Can you work these out from the model? Positions are in its coordinate system, mm. A direction names the side the tool comes from. Coordinates: 2 decimals unless noted, no trailing zeros. Order: outer loops, then holes, each group sorted by start corner. A loop starts at its lowest first (then second) coordinate and runs counter-clockwise, first axis right, second up. Notation, with made-up numbers: (59, -19) -> (98, -19) arc R22 cw to (98, -7) -> close; hole circle Ø11 at (17, 59). An arc over 180 degrees is marked (long way). Answer in a Markdown table with one row per item. Add a question column.
1. If I drill on line 1 along Y through (x, z) = (5.25, 2.7) (3 decimals); line 2 along Y through (x, z) = (5.75, 2.5); line 3 along X through (y, z) = (65, 2.45), over which ranges is the centre line in solid material (lowest first)? Write a range as [from, to].
2. On a 3-axis mill with a long thin cutter (end or side, diameter ignored), from which of +Z, -Z, +X, -X, +Y, -Y can I reach the whole of each face in a straight line? I mean faces 1 (the face through (7.561, 65.054, 3.507)), 2 (the face through (3.325, 14.513, 2.521)), 3 (the face through (6.8, 64.8, 2)), 4 (the face through (9.86, 13.47, 2.52)), 5 (the face through (6, 39, 4)). Say none if no direction works.
3. We'd pull the mould along X, two halves only. Please class faces 6 (the face through (3.29, 68.42, 3.51)), 7 (the face through (6, 39, 1)), 8 (the face through (11.116, 37.836, 2.479)), 9 (the face through (-0.461, 62.927, 2.521)): pulls with the +X half, pulls with the -X half, needs draft (parallel to the pull), parting line crosses it, or undercut.
4. Imagine slicing it at B-B on y = 50. Write out the boundary of the cut face in (x, z), plus the area to 3 significant figures.
5. Will these pins go through, and if not, where does the flat tip stop? pin 1 (4.5 mm diameter, centred on x = 5.59, y = 11.38, fed in from +Z); pin 2 (1.5 mm diameter, centred on x = 3, y = 43, fed in from -Z); pin 3 (1 mm diameter, centred on x = 2, z = 2, fed in from -Y).
6. Imagine slicing it at A-A on z = 1.55. Write out the boundary of the cut face in (x, y), plus the area to 3 significant figures.
7. Imagine slicing it at C-C on x = 10.5. Write out the boundary of the cut face in (y, z), plus the area to 3 significant figures.
Autodesk Inventor part; units mm, degrees
ref_plane "Work Plane1" through (-0.0405, 69.8618, 0) normal (0, 0, 1) x (0.6413599, 0.7672402, 0)
ref_plane "Work Plane3" through (5.5931, 11.378, 1) normal (0, 0, 1) x (1, 0, 0)
ref_plane "Work Plane6" through (4.3681, 64.2214, 5) normal (0, 0, 1) x (1, 0, 0)
ref_plane "Work Plane1" through (-0.0405, 69.8618, 0) normal (0, 0, 1) x (0.6413599, 0.7672402, 0)
ref_plane "Work Plane3" through (5.5931, 11.378, 1) normal (0, 0, 1) x (1, 0, 0)
sketch "Sketch2" plane through (5.5931, 11.378, 1) normal (0, 0, 1) x (1, 0, 0)
  arc A0 (-2.9323, 0.6339) -> (-4.1247, 52.0744) centre (-110.4489, 23.8756) ccw
  arc A1 (2.9323, -0.6339) -> (1.6748, 53.6125) centre (-110.4489, 23.8756) ccw
  arc A2 (1.6748, 53.6125) -> (-4.1247, 52.0744) centre (-1.225, 52.8435) ccw
  circle A3 centre (0, 0) radius 3
  circle A4 centre (0, 0) radius 1.25
  circle A5 centre (-1.225, 52.8435) radius 3
  circle A6 centre (-1.225, 52.8435) radius 1.4795
  point P0 (-5.5931, -11.378)
  point P1 (-2.9323, 0.6339)
  point P2 (2.9323, -0.6339)
extrude "Extrusion2" add sketch "Sketch2" along normal blind 3
ref_plane "Work Plane6" through (4.3681, 64.2214, 5) normal (0, 0, 1) x (1, 0, 0)
sketch "Sketch4" plane through (4.3681, 64.2214, 4) normal (0, 0, 1) x (1, 0, 0)
  arc A0 (4.1572, -53.4773) -> (2.8997, 0.7691) centre (-109.2239, -28.9678) ccw construction
  arc A1 (-1.7073, -52.2096) -> (-2.8997, -0.7691) centre (-109.2239, -28.9678) ccw construction
  circle A2 centre (0, 0) radius 3 construction
  circle A3 centre (0, 0) radius 3 construction
  circle A4 centre (0, 0) radius 1.4795 construction
  arc A5 (0.2521, -0.9677) -> (-0.2606, 0.9654) centre (-109.2239, -28.9678) ccw construction
  arc A6 (5.0961, 0.2712) -> (4.5608, 2.2899) centre (-109.2239, -28.9678) ccw
  arc A7 (-4.592, -2.2067) -> (-5.082, -0.359) centre (-109.2239, -28.9678) ccw
  arc A8 (-4.592, -2.2067) -> (5.0961, 0.2712) centre (0.2521, -0.9677) ccw
  arc A9 (4.5608, 2.2899) -> (-5.082, -0.359) centre (-0.2606, 0.9654) ccw
  arc A10 (-1.7073, -52.2096) -> (4.1572, -53.4773) centre (1.225, -52.8435) ccw
  arc A11 (2.8997, 0.7691) -> (-2.8997, -0.7691) centre (0, 0) ccw
  arc A12 (-1.7073, -52.2096) -> (-2.8997, -0.7691) centre (-109.2239, -28.9678) ccw
  point P0 (-4.3681, -64.2214)
  dimension "d16" = 10
  dimension "d26" = 1
  dimension "d27" = 1
extrude "Extrusion4" add sketch "Sketch4" against normal blind 3
ref_plane "Work Plane7" through (5.5931, 11.378, 5) normal (0, 0, 1) x (1, 0, 0)
sketch "Sketch5" plane through (5.5931, 11.378, 5) normal (0, 0, 1) x (1, 0, 0)
  arc A0 (-0.9646, 51.8435) -> (-1.4951, 53.8435) centre (-110.4489, 23.8756) ccw construction
  arc A1 (0.7309, 52.2766) -> (0.1923, 54.3076) centre (-110.4489, 23.8756) ccw
  arc A2 (-2.6602, 51.4103) -> (-3.1824, 53.3794) centre (-110.4489, 23.8756) ccw
  arc A3 (-2.6602, 51.4103) -> (0.7309, 52.2766) centre (-0.9646, 51.8435) ccw
  arc A4 (0.1923, 54.3076) -> (-3.1824, 53.3794) centre (-1.4951, 53.8435) ccw
  arc A5 (2.6687, 52.7716) -> (2.1206, 54.838) centre (-110.4489, 23.8756) ccw
  arc A6 (2.1206, 54.838) -> (-5.1108, 52.849) centre (-1.4951, 53.8435) ccw
  arc A7 (-4.598, 50.9153) -> (-5.1108, 52.849) centre (-110.4489, 23.8756) ccw
  arc A8 (-4.598, 50.9153) -> (2.6687, 52.7716) centre (-0.9646, 51.8435) ccw
  arc A9 (3.3358, 55.1334) -> (-6.307, 52.4844) centre (-1.4856, 53.8089) ccw
  arc A10 (3.8712, 53.1147) -> (3.3358, 55.1334) centre (-110.4489, 23.8756) ccw
  arc A11 (2.869, 48.6758) -> (3.8712, 53.1147) centre (-0.9729, 51.8758) ccw
  arc A12 (-5.817, 50.6368) -> (-2.9702, 47.292) centre (-0.9729, 51.8758) ccw
  arc A13 (-5.817, 50.6368) -> (-6.307, 52.4844) centre (-110.4489, 23.8756) ccw
  point P0 (-5.5931, -11.378)
  dimension "d12" = 3.5
extrude "Extrusion5" cut sketch "Sketch5" against normal blind 5 contours A3 A2 A4 A1
sketch "Sketch7" plane through (5.5931, 11.378, 4) normal (0, 0, 1) x (1, 0, 0)
  circle A0 centre (0, 0) radius 1.25
  circle A1 centre (0, 0) radius 1.8
  arc A2 (-3.9097, 0.8452) -> (3.9097, -0.8452) centre (0, 0) ccw
  arc A3 (4.2266, 0.621) -> (-3.5928, 2.3113) centre (0.3169, 1.4661) ccw
  arc A4 (-2.9323, 0.6339) -> (-2.9702, 47.292) centre (-110.4489, 23.8756) ccw
  arc A5 (2.9323, -0.6339) -> (2.869, 48.6758) centre (-110.4489, 23.8756) ccw
  line L0 (0.3169, 1.4661) -> (0, 0) construction
  line L1 (-3.5928, 2.3113) -> (-3.9097, 0.8452)
  line L2 (4.2266, 0.621) -> (3.9097, -0.8452)
  line L3 (-2.9323, 0.6339) -> (2.9323, -0.6339) construction
  point P0 (-5.5931, -11.378)
  dimension "d19" = 3.6
  dimension "d20" = 8
  dimension "d21" = 1.5
extrude "Extrusion6" cut sketch "Sketch7" against normal up to surface (3 mm away) contours A1
extrude "Extrusion7" add sketch "Sketch7" against normal up to surface (3 mm away) contours L1 A3 L2 A2
sketch "Sketch8" plane through (5.5931, 11.378, 4) normal (0, 0, 1) x (1, 0, 0)
  arc A0 (-2.6602, 51.4103) -> (-3.1824, 53.3794) centre (-110.4489, 23.8756) ccw
  arc A1 (0.1923, 54.3076) -> (-3.1824, 53.3794) centre (-1.4951, 53.8435) ccw
  arc A2 (0.7309, 52.2766) -> (0.1923, 54.3076) centre (-110.4489, 23.8756) ccw
  arc A3 (-2.6602, 51.4103) -> (0.7309, 52.2766) centre (-0.9646, 51.8435) ccw
  arc A4 (-3.3868, 51.2247) -> (-3.9056, 53.1805) centre (-110.4489, 23.8756) ccw
  arc A5 (-3.3868, 51.2247) -> (1.4576, 52.4622) centre (-0.9646, 51.8435) ccw
  arc A6 (1.4576, 52.4622) -> (0.9154, 54.5065) centre (-110.4489, 23.8756) ccw
  arc A7 (0.9154, 54.5065) -> (-3.9056, 53.1805) centre (-1.4951, 53.8435) ccw
  arc A8 (-4.162, 51.0267) -> (-4.6769, 52.9683) centre (-110.4489, 23.8756) ccw
  arc A9 (-4.162, 51.0267) -> (2.2327, 52.6602) centre (-0.9646, 51.8435) ccw
  arc A10 (2.2327, 52.6602) -> (1.6867, 54.7186) centre (-110.4489, 23.8756) ccw
  arc A11 (1.6867, 54.7186) -> (-4.6769, 52.9683) centre (-1.4951, 53.8435) ccw
  point P0 (-5.5931, -11.378)
  dimension "d31" = 2.5
  dimension "d32" = 0.8
extrude "Extrusion8" cut sketch "Sketch8" against normal up to surface (3 mm away) contours A4 A7 A6 A5
extrude "Extrusion9" cut sketch "Sketch8" against normal blind 1 contours A8 A11 A10 A9
sketch "Sketch9" plane through (5.5931, 11.378, 4) normal (0, 0, 1) x (1, 0, 0)
  arc A0 (-3.9097, 0.8452) -> (3.9097, -0.8452) centre (0, 0) ccw
  arc A1 (3.7507, 3.5177) -> (2.869, 48.6758) centre (-110.4489, 23.8756) ccw
  arc A2 (-4.162, 51.0267) -> (-4.6769, 52.9683) centre (-110.4489, 23.8756) ccw
  arc A3 (1.6867, 54.7186) -> (-4.6769, 52.9683) centre (-1.4951, 53.8435) ccw
  arc A4 (2.2327, 52.6602) -> (1.6867, 54.7186) centre (-110.4489, 23.8756) ccw
  arc A5 (-4.162, 51.0267) -> (2.2327, 52.6602) centre (-0.9646, 51.8435) ccw
  circle A6 centre (0, 0) radius 1.8
  arc A7 (3.7507, 3.5177) -> (2.869, 48.6758) centre (-110.4489, 23.8756) ccw
  arc A8 (2.869, 48.6758) -> (3.8712, 53.1147) centre (-0.9729, 51.8758) ccw
  arc A9 (3.8712, 53.1147) -> (3.3358, 55.1334) centre (-110.4489, 23.8756) ccw
  arc A10 (3.3358, 55.1334) -> (-6.307, 52.4844) centre (-1.4856, 53.8089) ccw
  arc A11 (-5.817, 50.6368) -> (-6.307, 52.4844) centre (-110.4489, 23.8756) ccw
  arc A12 (-5.817, 50.6368) -> (-2.9702, 47.292) centre (-0.9729, 51.8758) ccw
  arc A13 (-2.148, 4.6164) -> (-2.9702, 47.292) centre (-110.4489, 23.8756) ccw
  arc A14 (-2.148, 4.6164) -> (-3.5928, 2.3113) centre (0.3169, 1.4661) ccw
  line L0 (-3.5928, 2.3113) -> (-3.9097, 0.8452)
  arc A15 (-3.9097, 0.8452) -> (3.9097, -0.8452) centre (0, 0) ccw
  line L1 (3.9097, -0.8452) -> (4.2266, 0.621)
  arc A16 (4.2266, 0.621) -> (3.7507, 3.5177) centre (0.3169, 1.4661) ccw
  arc A17 (-3.7092, 1.1941) -> (-3.9097, 0.8452) centre (-3.262, 0.7051) ccw
  arc A18 (-3.7092, 1.1941) -> (-1.652, 5.5427) centre (-7.9997, 5.8848) ccw
  arc A19 (-2.148, 4.6164) -> (-2.9702, 47.292) centre (-110.4489, 23.8756) ccw
  arc A20 (-1.162, 11.3705) -> (-1.652, 5.5427) centre (95.5412, 0.3052) ccw
  point P0 (-5.5931, -11.378)
  point P1 (3.7507, 3.5177)
  point P2 (-1.162, 11.3705)
extrude "Extrusion10" cut sketch "Sketch9" against normal up to surface (3 mm away) contours L0 A14 A13 A20 A18 A17
Answers follow:
| question | item | result |
|---|---|---|
| 1 | line 1 | y = [7.393, 9.611], [13.145, 60.8], [67.44, 70.055] |
| 1 | line 2 | y = [7.38, 9.58], [13.17, 60.99], [67.1, 69.91] |
| 1 | line 3 | x = [-0.89, 1.61], [6.75, 9.33] |
| 2 | face 1 | +Z |
| 2 | face 2 | +Z, -Z, -X |
| 2 | face 3 | +Z, -Z |
| 2 | face 4 | +Z, -Z, +X |
| 2 | face 5 | +Z, +X, -X, +Y, -Y |
| 3 | face 6 | undercut |
| 3 | face 7 | needs draft |
| 3 | face 8 | pulls with the +X half |
| 3 | face 9 | pulls with the -X half |
| 4 | outline | (4.15, 1) -> (10.2, 1) -> (10.2, 4) -> (4.15, 4) -> close |
| 4 | area | 18.2 mm² |
| 5 | pin 1 | stops at z = 4 |
| 5 | pin 2 | passes through |
| 5 | pin 3 | stops at y = 8.84 |
| 6 | outline | (-0.71, 63.86) arc R108.46 cw to (-0.22, 62.01) arc R5 ccw to (2.62, 58.67) arc R110 cw to (4.43, 22.75) arc R97.33 ccw to (3.94, 16.92) arc R6.36 cw to (1.88, 12.57) arc R0.66 ccw to (1.68, 12.22) arc R4 ccw to (9.5, 10.53) -> (9.82, 12) arc R4 ccw to (9.34, 14.9) arc R116 ccw to (8.46, 60.05) arc R5 ccw to (9.46, 64.49) arc R119.11 ccw to (8.93, 66.51) arc R5 ccw to start; hole (1.69, 64.56) arc R109.72 cw to (2.21, 62.6) arc R2.5 ccw to (7.05, 63.84) arc R115.55 ccw to (6.51, 65.88) arc R2.5 ccw to start; hole circle Ø3.6 at (5.59, 11.38) |
| 6 | area | 373 mm² |
| 7 | outline | (23.04, 1) -> (47.46, 1) -> (47.46, 4) -> (23.04, 4) -> close |
| 7 | area | 73.3 mm² |
